from build123d import *


with BuildPart() as f3:
    # F3: sweep along a path in F2
    with BuildLine(Plane.XZ.offset(105.8403934839)) as f3_path:
        Line((-38.3972818889, 0), (-38.3972818889, 1000))
    # F0 (on Top) → F3 (sweep)
    with BuildSketch(Plane.XY):
        with BuildLine():
            Line((-38.3972818889, -105.8403934839), (0, 0))
            Line((0, 0), (-115.8749862256, 178.1249802876))
            Line((-115.8749862256, 178.1249802876), (-195.8749862256, 178.1249802876))
            Line((-195.8749862256, 178.1249802876), (-195.8749862256, 118.1249802876))
            Line((-195.8749862256, 118.1249802876), (-183.8749862256, 118.1249802876))
            ThreePointArc((-183.8749862256, 118.1249802876), (-169.8161117226, 84.1838547906), (-135.8749862256, 70.1249802876))
            Line((-135.8749862256, 70.1249802876), (-135.8749862256, 58.1249802876))
            Line((-135.8749862256, 58.1249802876), (-123.8749862256, 58.1249802876))
            ThreePointArc((-123.8749862256, 58.1249802876), (-101.2227507064, -34.329172857), (-38.3972818889, -105.8403934839))
        make_face()
    sweep(path=f3_path.line)


solid = f3.part
Model file for the job. Use its own axes, mm. Give positions to 0.01 mm unless a question says otherwise; leave off trailing zeros. Order: outer loops, then holes, each group sorted by start corner. A loop starts at its lowest first (then second) coordinate and runs counter-clockwise, first axis right, second up. Notation, with made-up numbers: (69.25, 50.25) -> (114.25, 50.25) arc R32 cw to (114.25, 76.25) -> close; hole circle Ø11 at (18, -31). An arc over 180 degrees is marked (long way). Use CSV: the item, a comma, the result in double quotes.
1. Band-saw the part on B-B, the plane y = 16. Give the cut face in (x, z).
Outcome:
outline,"(-119.39, 0) -> (-10.41, 0) -> (-10.41, 1000) -> (-119.39, 1000) -> close"
2. Band-saw the part on C-C, the plane x = -149. Give the cut face in (y, z).
Outcome:
outline,"(71.95, 0) -> (178.12, 0) -> (178.12, 1000) -> (71.95, 1000) -> close"
3. Band-saw the part on A-A, the plane z = 308.5. Give the cut face in (x, y), then the cut area to 3 significant figures.
Outcome:
outline,"(-195.87, 118.12) -> (-183.87, 118.12) arc R48 ccw to (-135.87, 70.12) -> (-135.87, 58.12) -> (-123.87, 58.12) arc R200 ccw to (-38.4, -105.84) -> (0, 0) -> (-115.87, 178.12) -> (-195.87, 178.12) -> close"
area,"25,500 mm²"
4. Drill centre lines: line 1 along Y through (x, z) = (-125, 613); line 2 along Y through (x, z) = (-58, 895.5); line 3 along X through (y, z) = (53, 197.5). Where is each one in solid material? Low to high. Write a range as from..to.
Outcome:
line 1,"58.12..178.12"
line 2,"-90.23..89.16"
line 3,"-123.81..-34.48"
5. Drop flat-ended pins along their axis: pin 1 (3.5 mm diameter, centred on x = -191.5, z = 252.5, fed in from -Y) (3 decimals); pin 2 (13 mm diameter, centred on y = 63.5, z = 701.5, fed in from -X) (3 decimals); pin 3 (5 mm diameter, centred on x = -69.5, y = -23, fed in from -Z); pin 4 (12 mm diameter, centred on y = 143, z = 352, fed in from +X). Give the stop position or say it passes through.
Outcome:
pin 1,"y = 118.125"
pin 2,"x = -135.875"
pin 3,"z = 0"
pin 4,"x = -89.12"
